Build history of the part. All positions in model axes, mm. A direction names the side the tool comes from. Coordinates: 2 decimals unless noted, no trailing zeros. Loops run counter-clockwise (first coordinate to the right, second up) from the corner with the lowest first, then second, coordinate; pieces in that order, holes last.
Item 1: Flat gauge pin, fed straight in: pin 1 (11 mm diameter, centred on y = 24, z = 0, fed in from -X). Where does the tip first touch, or does it go through?
Item 2: Cut at C-C (z = 4.25). List the corners of the cut face in (x, y), and give its area (3 significant figures).
Item 3: Drill centre lines: line 1 along Z through (x, y) = (0.5, 24); line 2 along Z through (x, y) = (-1.15, 19); line 3 along Y through (x, z) = (2.2, -3). Where is each one in solid material? Low to high.
Item 4: Cut at A-A (y = 29). List the corners of the cut face in (x, z), and give its area (3 significant figures).
Item 5: Cut at B-B (x = 0.3). List the corners of the cut face in (y, z), and give its area (3 significant figures).
Item 6: Mould opens along Z. For faces 1 (the face through (0, 15, -15)), 2 (the face through (0.042, 16.798, 4.226)), 3 (the face through (0, 14, 15)) say: released by +Z, released by -Z, zero draft, split by the parting line, or undercut.
Item 7: Cut at D-D (z = 0). List the corners of the cut face in (x, y), and give its area (3 significant figures).
Item 8: 3-axis set-ups, long thin cutter, end or side, ignore diameter. For faces 4 (the face through (0.04, 16.75, -4.27)), 5 (the face through (0, 30, 0)): which of +Z, -Z, +X, -X, +Y, -Y reach the whole face in a straight line?
from build123d import *

# Parameters (mm, degrees)
EXTRUDE_1_DEPTH = 3


with BuildPart() as part:
    # Эскиз2 → Бобышка-Вытянуть1 (new, symmetric)
    with BuildSketch(Plane(origin=(0, 0, 0), x_dir=(0, 0, -1), z_dir=(1, 0, 0))):
        with BuildLine():
            Line((15, 5), (6, 5))
            Line((6, 5), (6, 15))
            Line((6, 15), (2.5, 18.545643943))
            ThreePointArc((2.5, 18.545643943), (0, 30), (-2.5, 18.545643943))
            Line((-2.5, 18.545643943), (-6, 15))
            Line((-6, 15), (-6, 5))
            Line((-6, 5), (-15, 5))
            Line((-15, 5), (-15, 24))
            ThreePointArc((-15, 24), (0, 39), (15, 24))
            Line((15, 24), (15, 5))
        make_face()
    extrude(amount=EXTRUDE_1_DEPTH, both=True)


solid = part.part
Filled sheet:
1. pin 1: passes through
2. outline: (-3, 16.77) - (3, 16.77) - (3, 19.76) - (-3, 19.76) - close; (-3, 28.24) - (3, 28.24) - (3, 38.39) - (-3, 38.39) - close
2. area: 78.9 mm2
3. line 1: z = -15 to -6, 6 to 15
3. line 2: z = -15 to -3.32, 3.32 to 15
3. line 3: y = 18.04 to 18.8, 29.2 to 38.7
4. outline: (-3, -14.14) - (3, -14.14) - (3, -3.32) - (-3, -3.32) - close; (-3, 3.32) - (3, 3.32) - (3, 14.14) - (-3, 14.14) - close
4. area: 130 mm2
5. outline: (5, -15) - (24, -15) arc R15 ccw to (24, 15) - (5, 15) - (5, 6) - (15, 6) - (18.55, 2.5) arc R6 cw (long way) to (18.55, -2.5) - (15, -6) - (5, -6) - close
5. area: 662 mm2
6. face 1: released by -Z
6. face 2: undercut
6. face 3: released by +Z
7. outline: (-3, 30) - (3, 30) - (3, 39) - (-3, 39) - close
7. area: 54.0 mm2
8. face 4: +X, -X, -Y
8. face 5: +X, -X
